Geometry: final body of the model. Coordinates: model frame, mm. Face numbers are marked on the shaded views. A direction names the side the tool comes from. Give positions to 0.01 mm unless a question says otherwise; leave off trailing zeros. Order: outer loops, then holes, each group sorted by start corner. A loop starts at its lowest first (then second) coordinate and runs counter-clockwise, first axis right, second up. Notation, with made-up numbers: (48, -38) - (57, -38) arc R26 cw to (57, -16) - close; hole circle Ø11 at (48, -26). An arc over 180 degrees is marked (long way). One line per item, written item: value.
```python
from build123d import *

# Parameters (mm, degrees)
F0_W     = 2
F0_H     = 20
F1_DEPTH = 30
F2_R     = 5
F3_DEPTH = 2
F4_R     = 5
F5_DEPTH = 2
F6_R     = 1
F7_R     = 3


with BuildPart() as f1:
    # F0 (on Right) → F1 (new body)
    with BuildSketch(Plane.YZ):
        with Locations((1, 10)):
            Rectangle(F0_W, F0_H)
    extrude(amount=F1_DEPTH)

    # F2 (on face) → F3 (cut)
    with BuildSketch(Plane(origin=(0, 2, 0), x_dir=(-1, 0, 0), z_dir=(0, 1, 0))):
        with Locations((-10, 10)):
            Circle(F2_R)
    extrude(amount=-F3_DEPTH, mode=Mode.SUBTRACT)

    # F4 (on face) → F5 (join)
    with BuildSketch(Plane.YZ.offset(30)):
        Polygon((0, 20), (0, 0), (30, 0), (30, 20), (10, 20), (10, 16), (5, 16), (5, 20), align=None)
        with Locations((20, 10)):
            Circle(F4_R, mode=Mode.SUBTRACT)
    extrude(amount=F5_DEPTH)

    # F6
    f6_edges = [f1.edges().sort_by_distance(p)[0] for p in [
        (30, 2, 10),
        (31, 30, 0),
        (0, 1, 20),
        (0, 1, 0),
        (31, 30, 20),
    ]]
    fillet(f6_edges, radius=F6_R)

    # F7
    f7_edges = [f1.edges().sort_by_distance(p)[0] for p in [
        (32, 0, 10),
    ]]
    fillet(f7_edges, radius=F7_R)


solid = f1.part
```
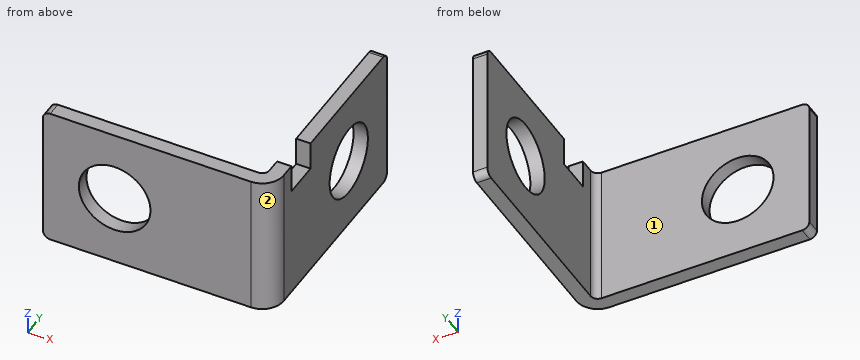
1) Section C-C, the plane y = 20. Return loops of the section in (x, z).
Answers below:
outline: (30, 0) - (32, 0) - (32, 5) - (30, 5) - close; (30, 15) - (32, 15) - (32, 20) - (30, 20) - close
2) First-contact query: pin 1 (1.6 mm diameter, centred on x = 30.5, z = 18.5, fed in from -Y); pin 2 (12 mm diameter, centred on x = 20.5, z = 9.5, fed in from +Y); pin 3 (3 mm diameter, centred on y = 13, z = 2.5, fed in from -X); pin 4 (12 mm diameter, centred on x = 27, z = 4, fed in from +Y). Flat tips, straight axial feed; report the tip coordinate or a pass-through.
Answers below:
pin 1: y = 0.08
pin 2: y = 2
pin 3: x = 30
pin 4: y = 30
3) Section B-B, the plane x = 10. Return loops of the section in (y, z).
Answers below:
outline: (0, 0) - (2, 0) - (2, 5) - (0, 5) - close; (0, 15) - (2, 15) - (2, 20) - (0, 20) - close
4) Section A-A, the plane z = 10. Return loops of the section in (x, y).
Answers below:
outline: (0, 0) - (5, 0) - (5, 2) - (0, 2) - close; (15, 0) - (29, 0) arc R3 ccw to (32, 3) - (32, 15) - (30, 15) - (30, 3) arc R1 cw to (29, 2) - (15, 2) - close; (30, 25) - (32, 25) - (32, 30) - (30, 30) - close
5) Set-up query: the marked faces 1 and 2. Return all of +Z, -Z, +X, -X, +Y, -Y with unobstructed straight access to the full face (end or side cutting, diameter ignored); none if empty.
Answers below:
face 1: +Z, -Z, -X, +Y
face 2: +Z, -Z, +X, -Y
6) Section D-D, the plane x = 25.5. Return loops of the section in (y, z).
Answers below:
outline: (0, 0) - (2, 0) - (2, 20) - (0, 20) - close
7) Material intervals for line 1 along Z through (x, y) = (10, 1.25); line 2 along Y through (x, z) = (22.5, 9.5); line 3 along X through (y, z) = (12, 2.75), sorted ascending.
Answers below:
line 1: 0 to 5, 15 to 20
line 2: 0 to 2
line 3: 30 to 32
